Geometry: see drawing. Coordinates: mm, zero at the bounding-box minimum. A direction names the side the tool comes from. Coordinates: 2 decimals unless noted, no trailing zeros. Loops run counter-clockwise (first coordinate to the right, second up) from the corner with the lowest first, then second, coordinate; pieces in that order, holes last. Notation, with made-up numbers: (80.25, 74) -> (120.25, 74) arc R28 ccw to (120.25, 104) -> close; hole circle Ø3 at (-15.75, 32). An arc over 180 degrees is marked (long way). Answer as a JSON object with one key per item and string values.
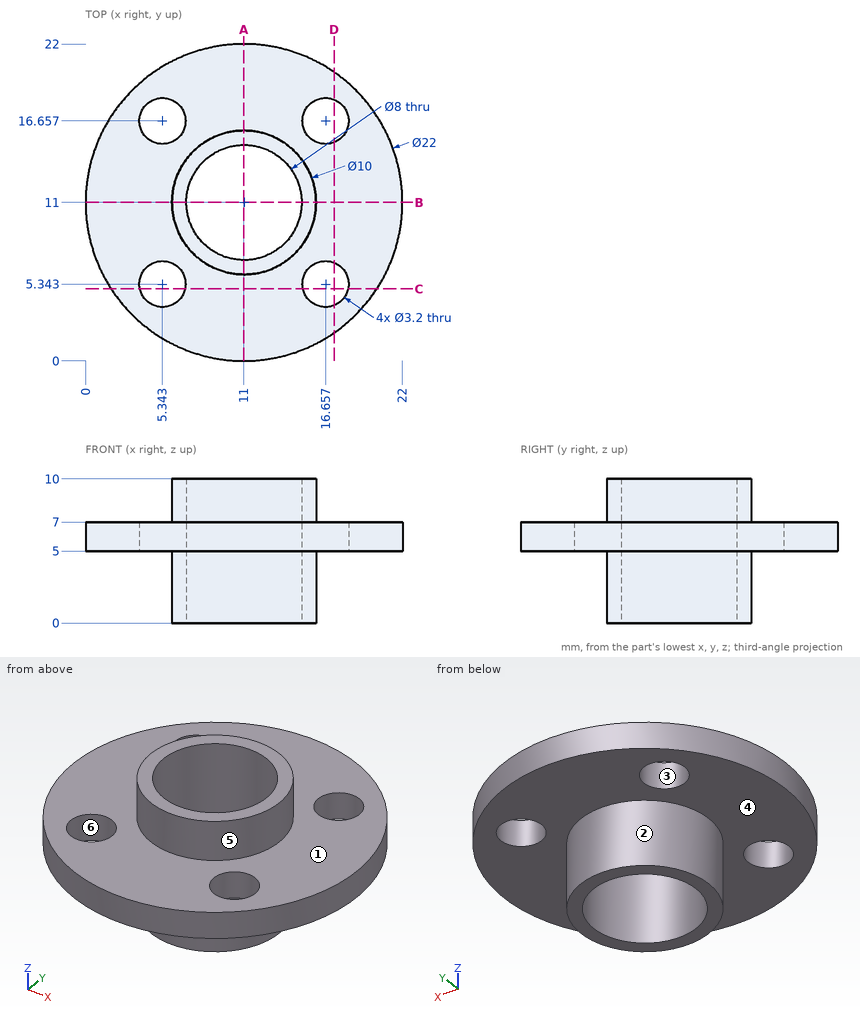
1. Section query A-A (x = 11). Return loops of the section in (y, z).
Reply:
{"outline": "(0, 5) -> (6, 5) -> (6, 0) -> (7, 0) -> (7, 10) -> (6, 10) -> (6, 7) -> (0, 7) -> close; (15, 0) -> (16, 0) -> (16, 5) -> (22, 5) -> (22, 7) -> (16, 7) -> (16, 10) -> (15, 10) -> close"}
2. Line query: line 1 along Z through (x, y) = (3.75, 10.75); line 2 along Y through (x, z) = (11, 4.25); line 3 along Y through (x, z) = (9.25, 4). Output: solid intervals per line, ascending.
Reply:
{"line 1": "z = 5 to 7", "line 2": "y = 6 to 7, 15 to 16", "line 3": "y = 6.32 to 7.4, 14.6 to 15.68"}
3. Pin query (flat end, axial travel): P1, Ø3, axis at x = 5.34, y = 16.66, coming from the +Z side; P2, Ø3.5, axis at x = 16.66, y = 5.34, coming from the -Z side; P3, Ø4, axis at x = 18, z = 6.5, coming from the -Y side; P4, Ø2, axis at x = 6.5, z = 6.5, coming from the +Y side. Return the tip coordinate at first contact, or that it passes through.
Reply:
{"P1": "passes through", "P2": "stops at z = 5", "P3": "stops at y = 1.2", "P4": "stops at y = 21.43"}
4. Access query for the marked faces 4, 5 and 6. Directions: +Z, -Z, +X, -X, +Y, -Y. A direction counts if a zero-diameter tool reaches every point of the face in a straight line with its end or side. Return the directions, or none.
Reply:
{"face 4": "-Z", "face 5": "+Z", "face 6": "+Z, -Z"}
5. Section query D-D (x = 17.25). Return loops of the section in (y, z), plus the area to 3 significant figures.
Reply:
{"outline": "(1.95, 5) -> (3.86, 5) -> (3.86, 7) -> (1.95, 7) -> close; (6.83, 5) -> (15.17, 5) -> (15.17, 7) -> (6.83, 7) -> close; (18.14, 5) -> (20.05, 5) -> (20.05, 7) -> (18.14, 7) -> close", "area": "24.3 mm2"}
6. Mould query, pull axis X, two halves, no side actions, for the marked faces 1, 2 and 3. Classes: pulls with the +X half, pulls with the -X half, needs draft (parallel to the pull), parting line crosses it, or undercut.
Reply:
{"face 1": "needs draft", "face 2": "parting line crosses it", "face 3": "undercut"}
7. Section query C-C (y = 5). Return loops of the section in (x, z).
Reply:
{"outline": "(1.78, 5) -> (3.78, 5) -> (3.78, 7) -> (1.78, 7) -> close; (6.91, 5) -> (15.09, 5) -> (15.09, 7) -> (6.91, 7) -> close; (18.22, 5) -> (20.22, 5) -> (20.22, 7) -> (18.22, 7) -> close"}
